```python
from build123d import *

# Parameters (mm, degrees)
SKETCH_W        = 457.2
SKETCH_H        = 31.75
PAD_DEPTH       = 25.4
SKETCH001_W     = 25.4
SKETCH001_H     = 6.35
POCKET_DEPTH    = 25.401
SKETCH002_W     = 25.4
SKETCH002_H     = 6.35
POCKET001_DEPTH = 25.401
SKETCH003_R     = 3.175
POCKET002_DEPTH = 31.751


with BuildPart() as part:
    # Sketch → Pad (new body)
    with BuildSketch(Plane.XZ):
        Rectangle(SKETCH_W, SKETCH_H)
    extrude(amount=PAD_DEPTH)

    # Sketch001 (on Face6 of Pad) → Pocket (cut, through all)
    with BuildSketch(Plane.XZ.offset(25.4)):
        with Locations((-215.9, 12.7)):
            Rectangle(SKETCH001_W, SKETCH001_H)
        with Locations((-215.9, 0)):
            Rectangle(SKETCH001_W, SKETCH001_H)
        with Locations((-215.9, -12.7)):
            Rectangle(SKETCH001_W, SKETCH001_H)
    extrude(amount=-POCKET_DEPTH, mode=Mode.SUBTRACT)

    # Sketch002 (on Face6 of Pad) → Pocket001 (cut, through all)
    with BuildSketch(Plane.XZ.offset(25.4)):
        with Locations((215.9, 6.35)):
            Rectangle(SKETCH002_W, SKETCH002_H)
        with Locations((215.9, -6.35)):
            Rectangle(SKETCH002_W, SKETCH002_H)
    extrude(amount=-POCKET001_DEPTH, mode=Mode.SUBTRACT)

    # Sketch003 (on Face21 of Pocket001) → Pocket002 (cut, through all)
    with BuildSketch(Plane(origin=(0, 0, 15.875), x_dir=(-1, 0, 0), z_dir=(0, 0, 1))):
        with Locations((215.9, 12.7)):
            Circle(SKETCH003_R)
        with Locations((-215.9, 12.7)):
            Circle(SKETCH003_R)
    extrude(amount=-POCKET002_DEPTH, mode=Mode.SUBTRACT)


solid = part.part
```
Check sheet for the modelled part. Datum: model origin and axes. Units: mm. A direction names the side the tool comes from. Round coordinates to 2 decimals unless told otherwise and drop trailing zeros. One line per item, written item: value. Start each with the question number.
Q1. Thickness scan on line 1 (Y direction, x = -215.9, z = -7) (3 decimals); line 2 (X direction, y = -12.7, z = 12.5) (3 decimals); line 3 (Y direction, x = 215, z = 0). Record the ranges inside material, lowest first.
Q2. Mould release check, pull along Z, two halves, no side actions. Record for faces 6 (the face through (10, -13, 15.875)), 7 (the face through (-3, -25.4, 0)), 8 (the face through (10, -13, -15.875)), 9 (the face through (-213, -10, -3.175)): pulls with the +Z half, pulls with the -Z half, needs draft (parallel to the pull), parting line crosses it, or undercut.
Q3. Gauge pin test, flat ends, axial feed: pin 1 Ø1.5 at (y, z) = (-10.5, 1.5) entering from -X; pin 2 Ø7.5 at (x, y) = (-221, -10.5) entering from +Z (3 decimals); pin 3 Ø5.5 at (x, y) = (-215.9, -12.7) entering from +Z; pin 4 Ø3 at (y, z) = (-19, -6) entering from +X. Record the tip position at first contact, or that the pin passes through.
Q4. Set-up check for faces 1 (the face through (-213, -10, 3.175)), 2 (the face through (219, -10, 9.525)), 3 (the face through (-213, -10, 9.525)), 4 (the face through (-213, -10, -9.525)), 5 (the face through (-3, 0, 0)): record each of +Z, -Z, +X, -X, +Y, -Y from which the full face is reachable in a straight line by a thin tool's end or side.
Completed:
1. line 1: y = -25.4 to -15.875, -9.525 to 0
1. line 2: x = -203.2 to 212.725, 219.075 to 228.6
1. line 3: y = -25.4 to -15.74, -9.66 to 0
2. face 6: pulls with the +Z half
2. face 7: needs draft
2. face 8: pulls with the -Z half
2. face 9: undercut
3. pin 1: stops at x = -203.2
3. pin 2: stops at z = 9.525
3. pin 3: passes through
3. pin 4: stops at x = 203.2
4. face 1: -X, +Y, -Y
4. face 2: +X, +Y, -Y
4. face 3: +Z, -X, +Y, -Y
4. face 4: -Z, -X, +Y, -Y
4. face 5: +Z, -Z, +X, -X, +Y
